Source: CAD feature listing. Evaluate the final solid. Frame: model axes, mm. Face numbers are marked on the shaded views. A direction names the side the tool comes from. Round coordinates to 2 decimals unless told otherwise and drop trailing zeros. Order: outer loops, then holes, each group sorted by start corner. A loop starts at its lowest first (then second) coordinate and runs counter-clockwise, first axis right, second up. Notation, with made-up numbers: (-12, 3.25) -> (20, 3.25) arc R18 cw to (20, 14.25) -> close; hole circle Ø6 at (17, 28.25). An arc over 180 degrees is marked (long way). Write item = value, one per line. Start each with the question number.
(1) Contact query for flat-ended pins moving along their axis: pin 1 Ø5 at (x, z) = (7, 2) entering from -Y; pin 2 Ø4 at (x, z) = (-3.5, 1.5) entering from -Y; pin 3 Ø1 at (x, z) = (4.5, -7) entering from -Y. Output: stop coordinate, or through.
(2) Cut plane C-C on y = -14.25. Return the cut outline in (x, z).
(3) Ray query, line 1 (Y direction, x = -5.75, z = 4.5); line 2 (X direction, y = -18.25, z = 0); line 3 (Y direction, x = 2, z = -4.75). Return the intervals inside material, ascending.
(4) Reachability of the marked faces 4 and 5 from +Z, -Z, +X, -X, +Y, -Y: full face, straight path, thin tool, end or side. Return the list, or none.
(5) Cut plane A-A on y = -11.5. Return the cut outline in (x, z).
(6) Cut plane B-B on z = -8. Return the cut outline in (x, y).
(7) Draft query along Y for the marked faces 1, 2 and 3. Return one class per face: released by +Y, released by -Y, zero draft, split by the parting line, or undercut.
from build123d import *

# Parameters (mm, degrees)
F0_R     = 9.525
F1_DEPTH = 6.35
F2_R     = 6.35
F3_DEPTH = 7.62
F4_R     = 7.62
F5_DEPTH = 7.62
F6_R     = 6.35


with BuildPart() as f1:
    # F0 (on Front) → F1 (new body)
    with BuildSketch(Plane.XZ):
        Circle(F0_R)
    extrude(amount=F1_DEPTH)

    # F2 (on face) → F3 (join)
    with BuildSketch(Plane.XZ.offset(6.35)):
        Circle(F2_R)
    extrude(amount=F3_DEPTH)

    # F4 (on face) → F5 (join)
    with BuildSketch(Plane.XZ.offset(13.97)):
        Circle(F4_R)
    extrude(amount=F5_DEPTH)

    # F6
    f6_edges = [f1.edges().sort_by_distance(p)[0] for p in [
        (-7.62, -21.59, 0),
    ]]
    fillet(f6_edges, radius=F6_R)


solid = f1.part
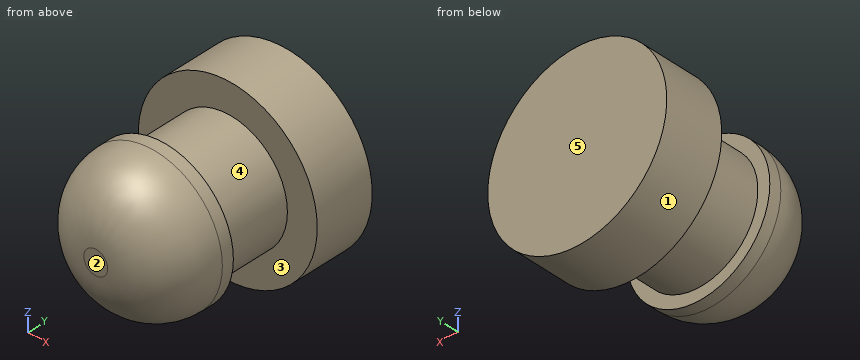
Evaluation:
q1.pin_1 = -20.53
q1.pin_2 = -21.57
q1.pin_3 = -6.35
q2.outline = circle Ø15.24 at (0, 0)
q3.line_1 = -17.23 to -13.97, -6.35 to 0
q3.line_2 = -6.86 to 6.86
q3.line_3 = -20.26 to 0
q4.face_4 = none
q4.face_5 = +Z, -Z, +X, -X, +Y
q5.outline = circle Ø12.7 at (0, 0)
q6.outline = (-5.17, -6.35) -> (5.17, -6.35) -> (5.17, 0) -> (-5.17, 0) -> close
q7.face_1 = zero draft
q7.face_2 = released by -Y
q7.face_3 = undercut
